Read the model definition and answer for the solid it produces. Units are mm, in the model's axes. Face numbers are marked on the shaded views. A direction names the side the tool comes from. Coordinates: 2 decimals unless noted, no trailing zeros. Write each loop counter-clockwise with the first axis right and the second up, starting at its lowest first coordinate (ties: lowest second). Pieces come first, ordered by that corner, then holes.
1) Determine the mould class of the marked faces 1, 2, 3 and 4 for opening direction Y: +Y half, -Y half, draft (parallel to the pull), parting line (faces both ways), or undercut.
2) The part is cut by section C-C (y = 7). Determine the outline of the cut face in (x, z), then the cut area to 3 significant figures.
3) Each of these flat-tipped pins is pushed along its axis until it touches: pin 1 Ø1 at (y, z) = (6.5, 0) entering from +X; pin 2 Ø3 at (x, y) = (-8.62, -6.65) entering from +Z; pin 3 Ø2 at (x, z) = (12.5, -0.5) entering from +Y. Where does it stop, or does it pass through?
4) The part is cut by section A-A (x = 0). Determine the outline of the cut face in (y, z).
5) The part is cut by section B-B (z = -1.2). Determine the outline of the cut face in (x, y).
6) Which of the six approach directions +Z, -Z, +X, -X, +Y, -Y give full straight-line access (tool end or side, diameter ignored) to the marked faces 5, 6, 7, 8 and 9?
7) The part is cut by section D-D (z = 2.1). Determine the outline of the cut face in (x, y), then the cut area to 3 significant figures.
8) Find the intervals of material crossed by line 1 (X direction, y = -7, z = 2.05); line 2 (Y direction, x = 0, z = -0.55); line 3 (Z direction, x = 0.5, y = -7.5), in increasing order.
Autodesk Inventor part; units mm, degrees
ref_plane "YZ Plane" through (0, 0, 0) normal (1, 0, 0) x (0, 1, 0)
ref_plane "XZ Plane" through (0, 0, 0) normal (0, 1, 0) x (-1, 0, 0)
ref_plane "XY Plane" through (0, 0, 0) normal (0, 0, 1) x (1, 0, 0)
sketch "Sketch1" plane through (0, 0, 0) normal (0, 0, 1) x (1, 0, 0)
  circle A0 centre (0, 0) radius 16
  dimension "d0" = 32
extrude "Extrusion1" add sketch "Sketch1" along normal blind 4
sketch "Sketch2" plane through (0, 0, 4) normal (0, 0, 1) x (1, 0, 0)
  circle A0 centre (0, 0) radius 16
  arc A1 (15.7569, -2.7784) -> (-15.7569, -2.7784) centre (0, 0) ccw
  line L0 (0, 0) -> (-15.7569, -2.7784) construction
  line L1 (0, 0) -> (16, 0) construction
  line L2 (0, 0) -> (15.7569, -2.7784) construction
  arc A2 (12.8025, -2.2574) -> (-12.8025, -2.2574) centre (0, 0) ccw
  line L3 (0, 0) -> (-12.8025, -2.2574) construction
  line L4 (0, 0) -> (13, 0) construction
  line L5 (0, 0) -> (12.8025, -2.2574) construction
  line L6 (-12.8025, -2.2574) -> (-15.7569, -2.7784)
  line L7 (12.8025, -2.2574) -> (15.7569, -2.7784)
  dimension "d3" = 170
  dimension "d4" = 160
  dimension "d5" = 13
  dimension "d6" = 170
  dimension "d7" = 160
extrude "Extrusion2" add sketch "Sketch2" along normal blind 2 and the other way blind 6 contours A0 L7 A2 L6 picked at (-14.8428, -1.3464)
sketch "Sketch3" plane through (0, 0, 6) normal (0, 0, 1) x (1, 0, 0)
  arc A0 (15.7569, -2.7784) -> (-15.7569, -2.7784) centre (0, 0) ccw
  line L0 (0, 16) -> (0, 18)
  circle A1 centre (0, 18) radius 2.5
  line L1 (-4.5077, 15.3519) -> (-5.0712, 17.2709)
  circle A2 centre (-5.0712, 17.2709) radius 2.5
  line L2 (-8.6503, 13.4601) -> (-9.7315, 15.1426)
  circle A3 centre (-9.7315, 15.1426) radius 2.5
  line L3 (-12.092, 10.4778) -> (-13.6035, 11.7875)
  circle A4 centre (-13.6035, 11.7875) radius 2.5
  line L4 (-14.5541, 6.6466) -> (-16.3734, 7.4775)
  circle A5 centre (-16.3734, 7.4775) radius 2.5
  line L5 (-15.8371, 2.277) -> (-17.8168, 2.5617)
  circle A6 centre (-17.8168, 2.5617) radius 2.5
  line L6 (-15.8371, -2.277) -> (-17.8168, -2.5617)
  circle A7 centre (-17.8168, -2.5617) radius 2.5
  line L7 (-14.5541, -6.6466) -> (-16.3734, -7.4775)
  circle A8 centre (-16.3734, -7.4775) radius 2.5
  line L8 (-12.092, -10.4778) -> (-13.6035, -11.7875)
  circle A9 centre (-13.6035, -11.7875) radius 2.5
  line L9 (-8.6503, -13.4601) -> (-9.7315, -15.1426)
  circle A10 centre (-9.7315, -15.1426) radius 2.5
  line L10 (-4.5077, -15.3519) -> (-5.0712, -17.2709)
  circle A11 centre (-5.0712, -17.2709) radius 2.5
  line L11 (0, -16) -> (0, -18)
  circle A12 centre (0, -18) radius 2.5
  line L12 (4.5077, -15.3519) -> (5.0712, -17.2709)
  circle A13 centre (5.0712, -17.2709) radius 2.5
  line L13 (8.6503, -13.4601) -> (9.7315, -15.1426)
  circle A14 centre (9.7315, -15.1426) radius 2.5
  line L14 (12.092, -10.4778) -> (13.6035, -11.7875)
  circle A15 centre (13.6035, -11.7875) radius 2.5
  line L15 (14.5541, -6.6466) -> (16.3734, -7.4775)
  circle A16 centre (16.3734, -7.4775) radius 2.5
  line L16 (15.8371, -2.277) -> (17.8168, -2.5617)
  circle A17 centre (17.8168, -2.5617) radius 2.5
  line L17 (15.8371, 2.277) -> (17.8168, 2.5617)
  circle A18 centre (17.8168, 2.5617) radius 2.5
  line L18 (14.5541, 6.6466) -> (16.3734, 7.4775)
  circle A19 centre (16.3734, 7.4775) radius 2.5
  line L19 (12.092, 10.4778) -> (13.6035, 11.7875)
  circle A20 centre (13.6035, 11.7875) radius 2.5
  line L20 (8.6503, 13.4601) -> (9.7315, 15.1426)
  circle A21 centre (9.7315, 15.1426) radius 2.5
  line L21 (4.5077, 15.3519) -> (5.0712, 17.2709)
  circle A22 centre (5.0712, 17.2709) radius 2.5
  dimension "d12" = 2
  dimension "d13" = 5
  dimension "d16" = 360
extrude "Extrusion3" cut sketch "Sketch3" against normal blind 9.25 contours A6 A0 | A0 A6 | A5 A0 | A0 A5 | A4 A0 | A0 A4 | A3 A0 | A0 A3 | A2 A0 | A0 A2 | A1 A0 | A0 A1 | A22 A0 | A0 A22 | A21 A0 | A0 A21 | A20 A0 | A0 A20 | A19 A0 | A0 A19 | A18 A0 | A0 A18
sketch "Sketch4" plane through (0, 0, 4) normal (0, 0, 1) x (1, 0, 0)
  circle A0 centre (0, 0) radius 3.05
  dimension "d20" = 6.1
extrude "Extrusion4" cut sketch "Sketch4" along normal blind 9.25 and the other way blind 8.875
chamfer "Chamfer1" distance 2 angle 45 4 edges at (-14.2797, -2.5179, 6) (-14.2797, -2.5179, -2) (14.2797, -2.5179, 6) (14.2797, -2.5179, -2)
sketch "Sketch5" plane through (0, 0, 4) normal (0, 0, 1) x (1, 0, 0)
  line L0 (0, 0) -> (12.557, 3.3646)
  arc A0 (12.9974, -0.2609) -> (-12.9974, -0.2609) centre (0, 0) ccw
  line L1 (0, 0) -> (13, 0) construction
  line L2 (0, 0) -> (2.8978, 0.7765)
  circle A1 centre (0, 0) radius 3.05
  line L3 (0, 0) -> (1.4489, 0.3882)
  arc A2 (7.2444, 1.9411) -> (-4.3467, -1.1647) centre (1.4489, 0.3882) ccw
  line L4 (1.4489, 0.3882) -> (7.2444, 1.9411) construction
  line L5 (1.4489, 0.3882) -> (-4.3467, -1.1647) construction
  arc A3 (10.1422, 2.7176) -> (-7.2444, -1.9411) centre (1.4489, 0.3882) ccw
  line L6 (-7.2444, -1.9411) -> (-4.3467, -1.1647)
  line L7 (7.2444, 1.9411) -> (10.1422, 2.7176)
  dimension "d26" = 15
  dimension "d33" = 1.5
  dimension "d34" = 6
  dimension "d35" = 180
  dimension "d36" = 9
extrude "Extrusion5" add sketch "Sketch5" along normal blind 5 contours A2 L6 A3 L0
sketch "Sketch6" plane through (0, 0, 0) normal (0, 0, -1) x (-1, 0, 0)
  circle A0 centre (0, 0) radius 3
  circle A1 centre (0, 0) radius 6
  dimension "d38" = 12
extrude "Extrusion6" add sketch "Sketch6" along normal blind 2
sketch "Sketch7" plane through (0, 0, 4) normal (0, 0, 1) x (1, 0, 0)
  arc A0 (-15.9763, 0.8697) -> (-15.9806, -0.787) centre (0, 0) ccw
  arc A1 (15.9806, -0.787) -> (15.9763, 0.8697) centre (0, 0) ccw
  arc A2 (-15.9763, 0.8697) -> (15.9806, -0.787) centre (0, 0) ccw
  arc A3 (12.9974, -0.2609) -> (-12.9974, -0.2609) centre (0, 0) ccw
  arc A4 (-13, 0) -> (13, 0) centre (0, 0) ccw
  line L0 (0, 0) -> (13, 0) construction
  line L1 (0, 0) -> (-13, 0) construction
  line L2 (-15.9763, 0.8697) -> (-13, 0)
  line L3 (13, 0) -> (15.9763, 0.8697)
  dimension "d41" = 13
  dimension "d42" = 180
extrude "Extrusion7" add sketch "Sketch7" along normal blind 2 contours L2 A3 A4 L3 A1 A2 A0
sketch "Sketch12" plane through (0, 0, 4) normal (0, 0, 1) x (1, 0, 0)
  circle A0 centre (0, 0) radius 13
extrude "Extrusion11" add sketch "Sketch12" along normal blind 2
sketch "Sketch8" plane through (0, 0, 0) normal (0, 0, -1) x (-1, 0, 0)
  arc A0 (-6.62, -8.785) -> (7.502, -8.0449) centre (0, 0) ccw
  line L0 (0, 0) -> (-6.62, -8.785) construction
  line L1 (0, 0) -> (11, 0) construction
  line L2 (0, 0) -> (7.502, -8.0449) construction
  circle A1 centre (-6.62, -8.785) radius 2.5
  circle A2 centre (7.502, -8.0449) radius 2.5
  dimension "d45" = 11
  dimension "d46" = 127
  dimension "d47" = 80
  dimension "d48" = 5
  dimension "d49" = 5
extrude "Extrusion8" [suppressed]
sketch "Sketch13" plane through (0, 0, 6) normal (0, 0, 1) x (1, 0, 0)
  circle A0 centre (0, 0) radius 3.15
  dimension "d72" = 6.3
extrude "Extrusion12" cut sketch "Sketch13" against normal blind 10.25
sketch "Sketch14" plane through (0, 0, 6) normal (0, 0, 1) x (1, 0, 0)
  point P0 (0, 0)
sketch "Sketch15" plane through (0, 0, 6) normal (0, 0, 1) x (1, 0, 0)
  arc A0 (-8.6212, -6.6525) -> (8.1676, -8.1213) centre (0.3894, -0.3431) ccw
  line L0 (0.3894, -0.3431) -> (-8.6212, -6.6525) construction
  line L1 (0.3894, -0.3431) -> (11.3894, -0.3431) construction
  line L2 (0.3894, -0.3431) -> (8.1676, -8.1213) construction
  circle A1 centre (-8.6212, -6.6525) radius 2.55
  circle A2 centre (8.1676, -8.1213) radius 2.55
  point P0 (0, 0)
  dimension "d73" = 11
  dimension "d74" = 145
  dimension "d75" = 100
  dimension "d76" = 5.1
  dimension "d77" = 5.1
extrude "Extrusion13" cut sketch "Sketch15" against normal blind 5
fillet "Fillet6" radius 1.2 4 edges at (-7.2444, -1.9411, 7.5) (-4.3467, -1.1647, 7.5) (7.2444, 1.9411, 7.5) (10.1422, 2.7176, 7.5)
sketch "Sketch16" plane through (-8.6212, -6.6525, 1) normal (0, 0, 1) x (1, 0, 0)
  circle A0 centre (0, 0) radius 1
  circle A1 centre (16.7888, -1.4688) radius 2.55
  circle A2 centre (16.7888, -1.4688) radius 1
  point P0 (8.6212, 6.6525)
  dimension "d84" = 2
  dimension "d85" = 2
extrude "Extrusion14" [suppressed]
sketch "Sketch18" plane through (0, 0, 6) normal (0, 0, 1) x (1, 0, 0)
  arc A0 (-1.4128, 15.9375) -> (-3.1345, 15.69) centre (0, 0) ccw
  line L0 (-3.1345, 15.69) -> (-2.0992, 19.5537)
  line L1 (-3.1345, 15.69) -> (0.8655, 15.69) construction
  arc A1 (3.1345, 15.69) -> (1.4128, 15.9375) centre (0, 0) ccw
  arc A2 (3.1345, 15.69) -> (5.8457, 14.8939) centre (5.0712, 17.2709) ccw
  line L2 (3.1345, 15.69) -> (2.0992, 19.5537)
  line L3 (3.1345, 15.69) -> (7.1345, 15.69) construction
  line L4 (2.0992, 19.5537) -> (-2.0992, 19.5537)
  arc A3 (-5.8457, 14.8939) -> (-3.1345, 15.69) centre (-5.0712, 17.2709) ccw
  line L5 (-3.1345, 15.69) -> (0, 14.2283)
  line L6 (-3.1345, 15.69) -> (0.324, 15.69) construction
  line L7 (0, 14.2283) -> (3.1345, 15.69)
  dimension "d94" = 4
  dimension "d95" = 75
  dimension "d96" = 4
  dimension "d97" = 105
  dimension "d98" = 25
extrude "Extrusion16" [suppressed]
fillet "Fillet11" [suppressed]
sketch "Sketch20" plane through (0, 0, 6) normal (0, 0, 1) x (1, 0, 0)
  line L0 (-0.1809, 19.5537) -> (0.1809, 19.5537)
  arc A0 (-0.1809, 19.5537) -> (-2.5957, 17.7007) centre (-0.1809, 17.0537) ccw
  arc A1 (2.5957, 17.7007) -> (0.1809, 19.5537) centre (0.1809, 17.0537) ccw
  line L1 (-2.8685, 16.6827) -> (-2.5957, 17.7007)
  line L2 (2.5957, 17.7007) -> (2.8685, 16.6827)
  line L3 (-1.1298, 16.2169) -> (-0.8571, 17.2348)
  arc A2 (-0.1809, 17.7537) -> (-0.8571, 17.2348) centre (-0.1809, 17.0537) ccw
  line L4 (-0.1809, 17.7537) -> (0.1809, 17.7537)
  arc A3 (0.8571, 17.2348) -> (0.1809, 17.7537) centre (0.1809, 17.0537) ccw
  line L5 (0.8571, 17.2348) -> (1.1298, 16.2169)
  line L6 (-1.1298, 16.2169) -> (-1.6475, 14.285)
  line L7 (-1.6475, 14.285) -> (1.6475, 14.285)
  line L8 (1.6475, 14.285) -> (1.1298, 16.2169)
  point P0 (0, 0)
  dimension "d112" = 1.8
  dimension "d113" = 2
extrude "Extrusion18" [suppressed]
fillet "Fillet12" [suppressed]
sketch "Sketch21" plane through (0, 0, 9) normal (0, 0, 1) x (1, 0, 0)
  point P0 (0, 0)
ref_plane "Work Plane1" through (0, 0, 3) normal (0, 0, 1) x (1, 0, 0)
sketch "Sketch22" plane through (0, 0, 3) normal (0, 0, 1) x (1, 0, 0)
  circle A0 centre (0, 0) radius 17.3364
extrude "Extrusion19" cut sketch "Sketch22" along normal blind 10
properties part number "knob_bottom"
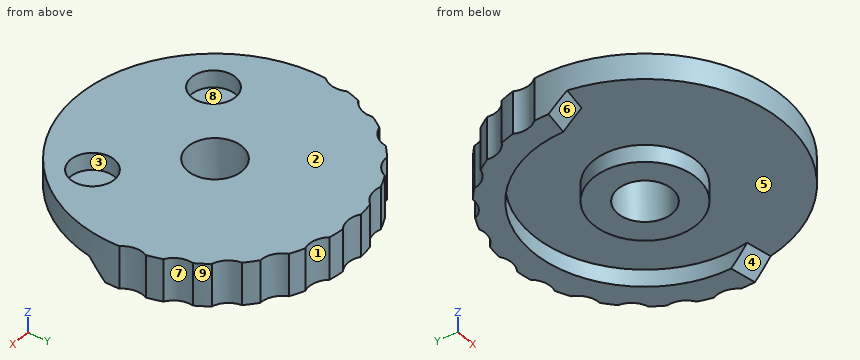
Reported:
1. face 1: +Y half
1. face 2: draft
1. face 3: undercut
1. face 4: -Y half
2. outline: (-13.92, -2) - (-10.95, -2) - (-10.95, 0) - (10.95, 0) - (10.95, -2) - (13.92, -2) - (13.92, 3) - (-13.92, 3) - close
2. area: 95.4 mm2
3. pin 1: stops at x = 14.36
3. pin 2: stops at z = 1
3. pin 3: stops at y = 10.44
4. outline: (-16, 0) - (-6, 0) - (-6, -2) - (-3.15, -2) - (-3.15, 3) - (-16, 3) - close; (3.15, -2) - (6, -2) - (6, 0) - (13, 0) - (13, -2) - (15.5, -2) - (15.5, 3) - (3.15, 3) - close
5. outline: (-15.98, 0.87) arc R16 ccw to (-15.92, -1.59) - (-12.96, -1.07) arc R13 cw (long way) to (12.96, -1.07) - (15.92, -1.59) arc R16 ccw to (15.98, 0.87) arc R2.5 cw to (15.57, 3.67) arc R16 ccw to (15.08, 5.34) arc R2.5 cw to (13.91, 7.91) arc R16 ccw to (12.97, 9.37) arc R2.5 cw to (11.12, 11.5) arc R16 ccw to (9.8, 12.64) arc R2.5 cw to (7.43, 14.17) arc R16 ccw to (5.85, 14.89) arc R2.5 cw to (3.13, 15.69) arc R16 ccw to (1.41, 15.94) arc R2.5 cw to (-1.41, 15.94) arc R16 ccw to (-3.13, 15.69) arc R2.5 cw to (-5.85, 14.89) arc R16 ccw to (-7.43, 14.17) arc R2.5 cw to (-9.8, 12.64) arc R16 ccw to (-11.12, 11.5) arc R2.5 cw to (-12.97, 9.37) arc R16 ccw to (-13.91, 7.91) arc R2.5 cw to (-15.08, 5.34) arc R16 ccw to (-15.57, 3.67) arc R2.5 cw to start; circle Ø12 at (0, 0); hole circle Ø6.3 at (0, 0)
6. face 5: -Z
6. face 6: -Z, -Y
6. face 7: +Z, -Z, +X
6. face 8: +Z
6. face 9: +Z, -Z, +X, +Y
7. outline: (-15.98, 0.87) arc R16 ccw (long way) to (15.98, 0.87) arc R2.5 cw to (15.57, 3.67) arc R16 ccw to (15.08, 5.34) arc R2.5 cw to (13.91, 7.91) arc R16 ccw to (12.97, 9.37) arc R2.5 cw to (11.12, 11.5) arc R16 ccw to (9.8, 12.64) arc R2.5 cw to (7.43, 14.17) arc R16 ccw to (5.85, 14.89) arc R2.5 cw to (3.13, 15.69) arc R16 ccw to (1.41, 15.94) arc R2.5 cw to (-1.41, 15.94) arc R16 ccw to (-3.13, 15.69) arc R2.5 cw to (-5.85, 14.89) arc R16 ccw to (-7.43, 14.17) arc R2.5 cw to (-9.8, 12.64) arc R16 ccw to (-11.12, 11.5) arc R2.5 cw to (-12.97, 9.37) arc R16 ccw to (-13.91, 7.91) arc R2.5 cw to (-15.08, 5.34) arc R16 ccw to (-15.57, 3.67) arc R2.5 cw to start; hole circle Ø5.1 at (-8.62, -6.65); hole circle Ø6.3 at (0, 0); hole circle Ø5.1 at (8.17, -8.12)
7. area: 722 mm2
8. line 1: x = -14.39 to -11.15, -6.09 to 5.88, 10.46 to 14.39
8. line 2: y = -6 to -3.15, 3.15 to 6, 13 to 15.5
8. line 3: z = 0 to 3
